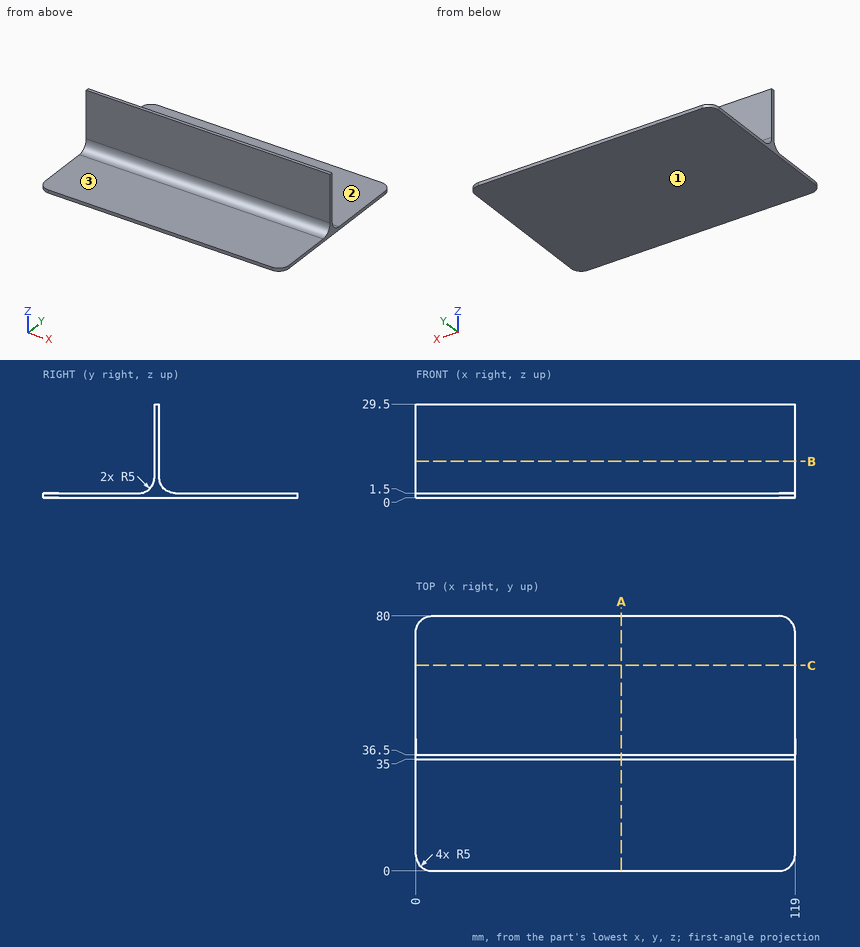
Print and shaded views of the part. All mm, measured from the part's lowest x, y and z. A direction names the side the tool comes from. Coordinates: 2 decimals unless noted, no trailing zeros. Write each loop counter-clockwise with the first axis right and the second up, starting at its lowest first coordinate (ties: lowest second). Pieces come first, ordered by that corner, then holes.
(1) Cut at A-A, the plane x = 64.5. List the corners of the cut face in (y, z).
(2) Drill centre lines: probe 1 along Z at (x, y) = (104, 20); probe 2 along Y at (x, z) = (37, 22.25); probe 3 along Z at (x, y) = (81, 34.5). Where is each one in solid material? Low to high.
(3) Cut at C-C, the plane y = 64.5. List the corners of the cut face in (x, z), and give its area (4 significant figures).
(4) Flat gauge pins, fed straight in: pin 1 (10 mm diameter, centred on x = 97, z = 21.5, fed in from -Y); pin 2 (12 mm diameter, centred on x = 20.5, z = 15, fed in from +Y); pin 3 (24 mm diameter, centred on x = 55.5, y = 14, fed in from +Z); pin 4 (1 mm diameter, centred on y = 38, z = 14, fed in from +X). Where does each tip first touch, or does it go through?
(5) Cut at B-B, the plane z = 11.5. List the corners of the cut face in (x, y).
(6) 3-axis set-ups, long thin cutter, end or side, ignore diameter. For the marked faces 1, 2 and 3: which of +Z, -Z, +X, -X, +Y, -Y reach the whole face in a straight line?
Geometry says:
1. outline: (0, 0) - (80, 0) - (80, 1.5) - (41.5, 1.5) arc R5 cw to (36.5, 6.5) - (36.5, 29.5) - (35, 29.5) - (35, 6.5) arc R5 cw to (30, 1.5) - (0, 1.5) - close
2. probe 1: z = 0 to 1.5
2. probe 2: y = 35 to 36.5
2. probe 3: z = 0 to 4.32
3. outline: (0, 0) - (119, 0) - (119, 1.5) - (0, 1.5) - close
3. area: 178.5 mm2
4. pin 1: stops at y = 35
4. pin 2: stops at y = 36.5
4. pin 3: stops at z = 1.5
4. pin 4: passes through
5. outline: (0, 35) - (119, 35) - (119, 36.5) - (0, 36.5) - close
6. face 1: -Z, +X, -X, +Y, -Y
6. face 2: +Z, +X, -X, +Y
6. face 3: +Z, +X, -X, -Y
